from build123d import *

# Parameters (mm, degrees)
F0_R     = 4.03124
F1_DEPTH = 4
F2_R     = 13.75
F3_DEPTH = 30
F4_R     = 3
F5_DEPTH = 12


# Not quite as in the source:
# - a feature names something its author has since deleted; it is built from what else it names


with BuildPart() as f1:
    # F0 (on Top) → F1 (new body)
    with BuildSketch(Plane.XY):
        Circle(F0_R)
    extrude(amount=F1_DEPTH)

    # F2 (on face) → F3 (join)
    with BuildSketch(Plane.XY.offset(4)):
        Circle(F2_R)
    extrude(amount=F3_DEPTH)

    # F4 (on face) → F5 (join)
    with BuildSketch(Plane.XY.offset(34)):
        Circle(F4_R)
    extrude(amount=F5_DEPTH)


solid = f1.part
The listing builds one solid part. Answer for the finished solid, in the listing's coordinates (mm). A direction names the side the tool comes from. Give positions to 0.01 mm unless a question says otherwise; leave off trailing zeros. Loops run counter-clockwise (first coordinate to the right, second up) from the corner with the lowest first, then second, coordinate; pieces in that order, holes last.
Item 1: A cutting plane is placed at D-D (x = 5.75). Give the vertices of the cut face in (y, z).
Derived:
outline: (-12.49, 4) - (12.49, 4) - (12.49, 34) - (-12.49, 34) - close
Item 2: Each of these flat-tipped pins is pushed along its axis until it touches: pin 1 Ø2 at (x, z) = (-2, 30) entering from -Y; pin 2 Ø4 at (x, y) = (9, 2) entering from -Z; pin 3 Ø1 at (x, z) = (-7, 13) entering from -Y; pin 4 Ø4 at (x, z) = (-5.5, 36.5) entering from +Y. Where does it stop, or does it pass through?
Derived:
pin 1: stops at y = -13.71
pin 2: stops at z = 4
pin 3: stops at y = -12.12
pin 4: passes through
Item 3: A cutting plane is placed at C-C (z = 27.5). Give the vertices of the cut face in (x, y), then the cut area to 3 significant figures.
Derived:
outline: circle Ø27.5 at (0, 0)
area: 594 mm2
Item 4: A cutting plane is placed at A-A (y = 0). Give the vertices of the cut face in (x, z), then the cut area to 3 significant figures.
Derived:
outline: (-13.75, 4) - (-4.03, 4) - (-4.03, 0) - (4.03, 0) - (4.03, 4) - (13.75, 4) - (13.75, 34) - (3, 34) - (3, 46) - (-3, 46) - (-3, 34) - (-13.75, 34) - close
area: 929 mm2
Item 5: Find the intervals of material crossed by line 1 along Z through (x, y) = (-9.5, 8.75); line 2 along Z through (x, y) = (2, 2.5); line 3 along Y through (x, z) = (-0.25, 19), in increasing order.
Derived:
line 1: z = 4 to 34
line 2: z = 0 to 34
line 3: y = -13.75 to 13.75
Item 6: A tool of negligible diameter and unlimited length cuts with its end or side. For faces 1 (the cylindrical face through (-3, 0, 40)), 2 (the cylindrical face through (-0.874, -3.935, 1.972)), 3 (the flat face through (0, 0, 46)), from which of +Z, -Z, +X, -X, +Y, -Y can it reach the whole face along a straight path? Write none if from no direction.
Derived:
face 1: +Z
face 2: -Z
face 3: +Z, +X, -X, +Y, -Y
